The model under review builds one solid part; all positions refer to its coordinate system, in mm. A direction names the side the tool comes from. Round coordinates to 2 decimals unless told otherwise and drop trailing zeros. Order: outer loops, then holes, each group sorted by start corner. A loop starts at its lowest first (then second) coordinate and runs counter-clockwise, first axis right, second up. Notation, with made-up numbers: (-16.5, 56.5) -> (1.5, 56.5) arc R16 ccw to (1.5, 75.5) -> close; hole circle Ø5 at (3.25, 86). An arc over 180 degrees is marked (long way). Use a Markdown table: item, result. Add a question column.
```python
from build123d import *

# Parameters (mm, degrees)
SKETCH_1_R          = 26
EXTRUDE_1_DEPTH     = 20
CUT_EXTRUDE_START   = -2
SKETCH_2_R          = 26
SKETCH_2_R_2        = 23
CUT_EXTRUDE_1_DEPTH = 16
SKETCH_3_R          = 5
CUT_EXTRUDE_2_DEPTH = 42.856899073
CHAMFER_1_SIZE      = 0.5
SKETCH_4_R          = 1.25
CUT_EXTRUDE_3_DEPTH = 42.856899073
SKETCH_5_R          = 1.25
CUT_EXTRUDE_4_DEPTH = 42.856899073


with BuildPart() as part:
    # 草图1 → 凸台-拉伸1 (new body)
    with BuildSketch(Plane(origin=(0, 0, 0), x_dir=(1, 0, 0), z_dir=(0, 1, 0))):
        with Locations(Location((0, 0, 0), (0, 0, 270))):
            Circle(SKETCH_1_R)
    extrude(amount=EXTRUDE_1_DEPTH)

    # 草图2 → 切除-拉伸1 (cut)
    with BuildSketch(Plane.XZ.offset(CUT_EXTRUDE_START)):
        with Locations(Location((0, 0, 0), (0, 0, 270))):
            Circle(SKETCH_2_R)
        with Locations(Location((0, 0, 0), (0, 0, 270))):
            Circle(SKETCH_2_R_2, mode=Mode.SUBTRACT)
    extrude(amount=-CUT_EXTRUDE_1_DEPTH, mode=Mode.SUBTRACT)

    # 草图3 → 切除-拉伸2 (cut, through all)
    with BuildSketch(Plane.XZ):
        with Locations(Location((0, 0, 0), (0, 0, 270))):
            Circle(SKETCH_3_R)
    extrude(amount=-CUT_EXTRUDE_2_DEPTH, mode=Mode.SUBTRACT)

    # 倒角1
    chamfer_1_edges = [part.edges().sort_by_distance(p)[0] for p in [
        (0, 20, 5),
        (0, 0, 5),
    ]]
    chamfer(chamfer_1_edges, length=CHAMFER_1_SIZE)

    # 草图4 → 切除-拉伸3 (cut, through all)
    with BuildSketch(Plane.XY):
        with Locations(Location((0, 10, 0), (0, 0, 90))):
            Circle(SKETCH_4_R)
    extrude(amount=-CUT_EXTRUDE_3_DEPTH, mode=Mode.SUBTRACT)

    # 草图5 → 切除-拉伸4 (cut, through all)
    with BuildSketch(Plane(origin=(0, 0, 0), x_dir=(0, 0, -1), z_dir=(1, 0, 0))):
        with Locations((0, 10)):
            Circle(SKETCH_5_R)
    extrude(amount=-CUT_EXTRUDE_4_DEPTH, mode=Mode.SUBTRACT)


solid = part.part
```
Q1. Add section D-D, the plane z = 17.5. Give the boundary of the cut face in (x, y), then the cut area to 3 significant figures.
Q2. Add section C-C, the plane y = 8. Give the boundary of the cut face in (x, z), then the cut area to 3 significant figures.
Q3. Add section B-B, the plane z = -20. Give the boundary of the cut face in (x, y), then the cut area to 3 significant figures.
Q4. For pin 1 (2 mm diameter, centred on x = 0, y = 10, fed in from +Z); pin 2 (4 mm diameter, centred on y = 10, z = 0, fed in from -X); pin 3 (2 mm diameter, centred on y = 14, z = 5.5, fed in from -X), all flat-tipped, find the tip position at first contact; note any pin that passes through.
Q5. For faces 4 (the face through (-13.79, 11.24, 0.16)), 5 (the face through (6, 0, 0)), 6 (the face through (-0.05, 8.75, -13.79)), 7 (the face through (-21, 18, -10)), list the 3-axis set-ups (+Z, -Z, +X, -X, +Y, -Y) from which the entire face can be reached by the end or side of a thin tool; tool diameter is ignored.
Q6. To check wall thickness, follow line 1 along Y through (x, z) = (-13, 0); line 2 along X through (y, z) = (13.5, 0); line 3 along Y through (x, z) = (23, -8). State the ranges of each line that lie inside material, in increasing order.
Q7. Draft analysis for pull direction X (two halves, no side actions). For faces 1 (the face through (19.394, 9.888, -12.365)), 2 (the face through (4, 10, -3)), 3 (the face through (6, 20, 0)), state which applies: released by +X, released by -X, zero draft, split by the parting line, or undercut.
Q8. Add section A-A, the plane x = 0. Give the boundary of the cut face in (y, z), then the cut area to 4 significant figures.
Return value:
| question | item | result |
|---|---|---|
| 1 | outline | (-19.23, 0) -> (19.23, 0) -> (19.23, 2) -> (14.92, 2) -> (14.92, 18) -> (19.23, 18) -> (19.23, 20) -> (-19.23, 20) -> (-19.23, 18) -> (-14.92, 18) -> (-14.92, 2) -> (-19.23, 2) -> close |
| 1 | area | 631 mm² |
| 2 | outline | circle Ø46 at (0, 0); hole circle Ø10 at (0, 0) |
| 2 | area | 1,580 mm² |
| 3 | outline | (-16.61, 0) -> (16.61, 0) -> (16.61, 2) -> (11.36, 2) -> (11.36, 18) -> (16.61, 18) -> (16.61, 20) -> (-16.61, 20) -> (-16.61, 18) -> (-11.36, 18) -> (-11.36, 2) -> (-16.61, 2) -> close; hole circle Ø2.5 at (0, 10) |
| 3 | area | 491 mm² |
| 4 | pin 1 | z = 23 |
| 4 | pin 2 | x = -23 |
| 4 | pin 3 | x = -22.56 |
| 5 | face 4 | -X |
| 5 | face 5 | +Z, -Z, +X, -X, -Y |
| 5 | face 6 | -Z |
| 5 | face 7 | none |
| 6 | line 1 | 0 to 8.75, 11.25 to 20 |
| 6 | line 2 | -23 to -5, 5 to 23 |
| 6 | line 3 | 0 to 2, 18 to 20 |
| 7 | face 1 | split by the parting line |
| 7 | face 2 | undercut |
| 7 | face 3 | zero draft |
| 8 | outline | (0, -26) -> (2, -26) -> (2, -23) -> (8.75, -23) -> (8.75, -5) -> (0.5, -5) -> (0, -5.5) -> close; (0, 5.5) -> (0.5, 5) -> (19.5, 5) -> (20, 5.5) -> (20, 26) -> (18, 26) -> (18, 23) -> (2, 23) -> (2, 26) -> (0, 26) -> close; (11.25, -23) -> (18, -23) -> (18, -26) -> (20, -26) -> (20, -5.5) -> (19.5, -5) -> (11.25, -5) -> close |
| 8 | area | 698.5 mm² |
